from build123d import *

# Parameters (mm, degrees)
F1_DEPTH = 11.938
F2_W     = 11.938
F2_H     = 19.431
F3_DEPTH = 152.4
F4_W     = 11.938
F4_H     = 76.2
F5_DEPTH = 11.938


with BuildPart() as f1:
    # F0 (on Top) → F1 (new body)
    with BuildSketch(Plane.XY):
        Polygon((-23.423575, 152.4), (-23.423575, 0), (-4.007815, 0), (-4.007815, 76.2), (7.960665, 76.2), (7.960665, 0), (27.376425, 0), (27.376425, 152.4), align=None)
    extrude(amount=F1_DEPTH)

    # F2 (on face) → F3 (join)
    with BuildSketch(Plane(origin=(0, 152.4, 0), x_dir=(-1, 0, 0), z_dir=(0, 1, 0))):
        with Locations((-1.976425, 21.6535)):
            Rectangle(F2_W, F2_H)
        with Locations((-1.976425, -9.7155)):
            Rectangle(F2_W, F2_H)
    extrude(amount=-F3_DEPTH)

    # F4 (on face) → F5 (join)
    with BuildSketch(Plane(origin=(0, 0, 11.938), x_dir=(1, 0, 0), z_dir=(0, 0, -1))):
        with Locations((1.976425, -38.1)):
            Rectangle(F4_W, F4_H)
    extrude(amount=F5_DEPTH)


solid = f1.part
Input: part model. Units: mm. Frame: model coordinates. A direction names the side the tool comes from. Coordinates: 2 decimals unless noted, no trailing zeros. Order: outer loops, then holes, each group sorted by start corner. A loop starts at its lowest first (then second) coordinate and runs counter-clockwise, first axis right, second up. Notation, with made-up numbers: M -40,-39.5 L -21,-39.5 A19 cw -21,-21.5 Z; hole C -17,80 d3. An arc over 180 degrees is marked long. Write item = value, one per line. Start each with the question number.
(1) First-contact query: P1, Ø8, axis at x = 13.5, y = 53.5, coming from the +Z side; P2, Ø6, axis at x = 19.5, y = 68.5, coming from the -Z side; P3, Ø4, axis at y = 39.5, z = 14, coming from the -X side; P4, Ø21.5, axis at x = 18.5, y = 94, coming from the +Z side. Flat tips, straight axial feed; report the tip coordinate or a pass-through.
(2) Line query: line 1 along X through (y, z) = (62.5, -11); line 2 along Z through (x, y) = (-13.5, 33). Output: solid intervals per line, ascending. Write a range as [from, to].
(3) Reachability of faces 1 (the flat face through (-14, 77, 11.938)), 2 (the flat face through (18, 77, 11.938)), 3 (the flat face through (2, 0, 6)), 4 (the flat face through (18, 77, 0)), 5 (the flat face through (-14, 77, 0)) from +Z, -Z, +X, -X, +Y, -Y: full face, straight path, thin tool, end or side. Return the list, or none.
(4) Section C-C on x = 19. Output: boundary loops of the cut face in (y, z), and give its area (3 significant figures).
(5) Section A-A on y = 73. Output: boundary loops of the cut face in (x, z), and give its area (3 significant figures).
(6) Section D-D on z = 26.5. Output: boundary loops of the cut face in (x, y).
(7) Section B-B on y = 139. Output: boundary loops of the cut face in (x, z).
Result set:
q1.P1 = 11.94
q1.P2 = 0
q1.P3 = -3.99
q1.P4 = 31.37
q2.line_1 = [-3.99, 7.95]
q2.line_2 = [0, 11.94]
q3.face_1 = +Z, -X, +Y, -Y
q3.face_2 = +Z, +X, +Y, -Y
q3.face_3 = +Z, -Z, +X, -X, -Y
q3.face_4 = -Z, +X, +Y, -Y
q3.face_5 = -Z, -X, +Y, -Y
q4.outline = M 0,0 L 152.4,0 L 152.4,11.94 L 0,11.94 Z
q4.area = 1,820 mm²
q5.outline = M -23.42,0 L -4.01,0 L -4.01,11.94 L -23.42,11.94 Z; M -3.99,-19.43 L 7.95,-19.43 L 7.95,31.37 L -3.99,31.37 Z; M 7.96,0 L 27.38,0 L 27.38,11.94 L 7.96,11.94 Z
q5.area = 1,070 mm²
q6.outline = M -3.99,0 L 7.95,0 L 7.95,152.4 L -3.99,152.4 Z
q7.outline = M -23.42,0 L -3.99,0 L -3.99,-19.43 L 7.95,-19.43 L 7.95,0 L 27.38,0 L 27.38,11.94 L 7.95,11.94 L 7.95,31.37 L -3.99,31.37 L -3.99,11.94 L -23.42,11.94 Z
